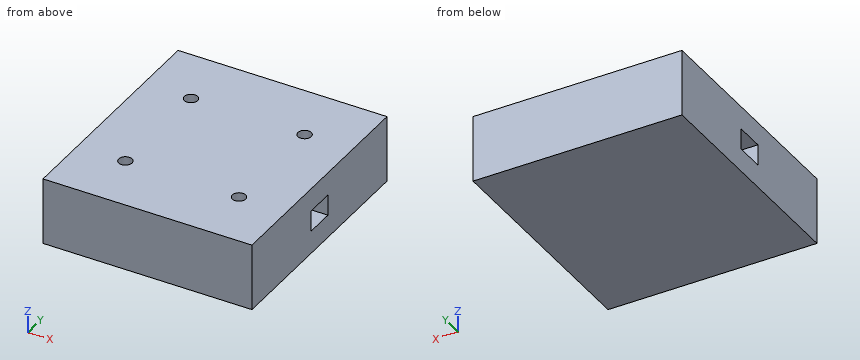
from build123d import *

# Parameters (mm, degrees)
F0_W     = 79.375
F0_H     = 25.4
F1_DEPTH = 88.9
F2_W     = 11.1125
F2_H     = 3.96875
F3_DEPTH = 19.05
F4_W     = 11.1125
F4_H     = 3.96875
F5_DEPTH = 19.05
F6_R     = 2.54
F7_DEPTH = 12.7


with BuildPart() as f1:
    # F0 (on Front) → F1 (new body)
    with BuildSketch(Plane.XZ):
        Rectangle(F0_W, F0_H)
    extrude(amount=F1_DEPTH)

    # F2 (on face) → F3 (cut)
    with BuildSketch(Plane.YZ.offset(39.6875)):
        with Locations((-44.45, -1.984375)):
            Rectangle(F2_W, F2_H)
        with Locations((-44.45, 1.984375)):
            Rectangle(F2_W, F2_H)
    extrude(amount=-F3_DEPTH, mode=Mode.SUBTRACT)

    # F4 (on face) → F5 (cut)
    with BuildSketch(Plane(origin=(-39.6875, 0, 0), x_dir=(0, -1, 0), z_dir=(-1, 0, 0))):
        with Locations((44.45, 1.984375)):
            Rectangle(F4_W, F4_H)
        with Locations((44.45, -1.984375)):
            Rectangle(F4_W, F4_H)
    extrude(amount=-F5_DEPTH, mode=Mode.SUBTRACT)

    # F6 (on face) → F7 (cut)
    with BuildSketch(Plane.XY.offset(12.7)):
        with Locations((-21.59, -22.86)):
            Circle(F6_R)
        with Locations((21.59, -22.86)):
            Circle(F6_R)
        with Locations((21.59, -66.04)):
            Circle(F6_R)
        with Locations((-21.59, -66.04)):
            Circle(F6_R)
    extrude(amount=-F7_DEPTH, mode=Mode.SUBTRACT)


solid = f1.part
Work out the finished part from the listing and answer in its coordinate system (mm). Round coordinates to 2 decimals unless told otherwise and drop trailing zeros. Write each loop counter-clockwise with the first axis right and the second up, starting at its lowest first coordinate (ties: lowest second). Pieces come first, ordered by that corner, then holes. Notation, with made-up numbers: (-29.5, 25.25) -> (-21.5, 25.25) arc R29 ccw to (-21.5, 53.25) -> close; hole circle Ø8 at (-17.5, -6.5). An arc over 180 degrees is marked (long way). Write each question's results on one line, items separated by ' | '.
Item 1: Flat-ended cylindrical pins translate along their axes: P1, Ø4, axis at y = -46.5, z = 0, coming from the -X side; P2, Ø4, axis at x = 21.5, y = -66.5, coming from the +Z side. Find the tip coordinate at first contact, or state that the pin passes through.
Result set:
P1: x = -20.64 | P2: z = 0
Item 2: A cutting plane is placed at B-B, the plane y = -66.04. Determine the outline of the cut face in (x, z).
Result set:
outline: (-39.69, -12.7) -> (39.69, -12.7) -> (39.69, 12.7) -> (24.13, 12.7) -> (24.13, 0) -> (19.05, 0) -> (19.05, 12.7) -> (-19.05, 12.7) -> (-19.05, 0) -> (-24.13, 0) -> (-24.13, 12.7) -> (-39.69, 12.7) -> close
Item 3: Find the intervals of material crossed by line 1 along Y through (x, z) = (-21.59, 6); line 2 along Z through (x, y) = (-33.5, -41.5); line 3 along X through (y, z) = (-45.5, -2), in increasing order. Write a range as [from, to].
Result set:
line 1: [-88.9, -68.58], [-63.5, -25.4], [-20.32, 0] | line 2: [-12.7, -3.97], [3.97, 12.7] | line 3: [-20.64, 20.64]
Item 4: A cutting plane is placed at A-A, the plane x = 27. Determine the outline of the cut face in (y, z).
Result set:
outline: (-88.9, -12.7) -> (0, -12.7) -> (0, 12.7) -> (-88.9, 12.7) -> close; hole (-50.01, -3.97) -> (-38.89, -3.97) -> (-38.89, 3.97) -> (-50.01, 3.97) -> close
